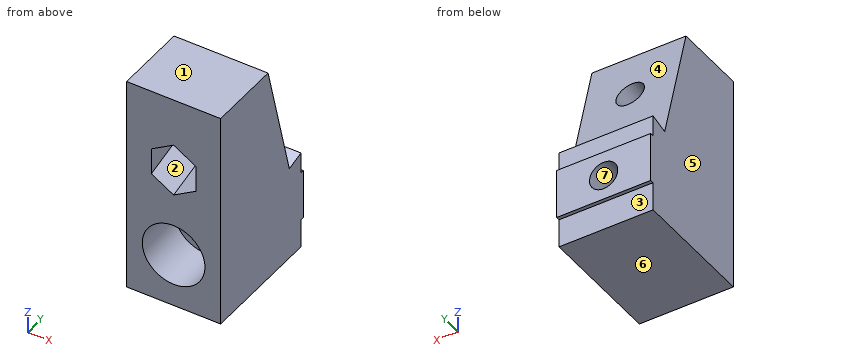
from build123d import *

# Parameters (mm, degrees)
BOSS_EXTRUDE1_DEPTH = 7.5
SKETCH2_R           = 2.25
CUT_EXTRUDE1_DEPTH  = 28.200078529
SKETCH3_R           = 2.25
CUT_EXTRUDE2_DEPTH  = 29.587584718
CUT_EXTRUDE3_START  = -4
CUT_EXTRUDE3_DEPTH  = 24.200078529
SKETCH5_W           = 15
SKETCH5_H           = 8
SKETCH5_R           = 2.25
BOSS_EXTRUDE2_DEPTH = 0.6
SKETCH6_R           = 5
CUT_EXTRUDE4_DEPTH  = 8


with BuildPart() as part:
    # Sketch1 → Boss-Extrude1 (new, symmetric)
    with BuildSketch(Plane(origin=(0, 0, 0), x_dir=(0, 0, -1), z_dir=(1, 0, 0))):
        Polygon((0.776457135, -2.897777479), (-19, -8.196863197), (-19, -20), (16, -20), (16, 0), (0, 0), align=None)
    extrude(amount=BOSS_EXTRUDE1_DEPTH, both=True)

    # Sketch2 → Cut-Extrude1 (cut, through all)
    with BuildSketch(Plane(origin=(0, -2.897777479, -0.776457135), x_dir=(1, 0, 0), z_dir=(0, 0.9659258262890682, 0.2588190451025216))):
        with Locations(Location((0, -12.003847577, 0), (0, 0, 270))):
            Circle(SKETCH2_R)
    extrude(amount=-CUT_EXTRUDE1_DEPTH, mode=Mode.SUBTRACT)

    # Sketch3 → Cut-Extrude2 (cut, through all)
    with BuildSketch(Plane.XZ.offset(20)):
        with Locations(Location((0, -7.39, 0), (0, 0, 270))):
            Circle(SKETCH3_R)
    extrude(amount=-CUT_EXTRUDE2_DEPTH, mode=Mode.SUBTRACT)

    # Sketch4 → Cut-Extrude3 (cut, through all)
    with BuildSketch(Plane(origin=(0, -2.897777479, -0.776457135), x_dir=(1, 0, 0), z_dir=(0, 0.9659258262890681, 0.2588190451025216)).offset(CUT_EXTRUDE3_START)):
        Polygon((0, -16.103034489), (3.55, -14.053441033), (3.55, -9.954254122), (0, -7.904660666), (-3.55, -9.954254122), (-3.55, -14.053441033), align=None)
    extrude(amount=-CUT_EXTRUDE3_DEPTH, mode=Mode.SUBTRACT)

    # Sketch5 → Boss-Extrude2 (add)
    with BuildSketch(Plane(origin=(0, 0, 0), x_dir=(1, 0, 0), z_dir=(0, 1, 0))):
        with Locations((0, 7.39)):
            Rectangle(SKETCH5_W, SKETCH5_H)
        with Locations(Location((0, 7.39, 0), (0, 0, 90))):
            Circle(SKETCH5_R, mode=Mode.SUBTRACT)
    extrude(amount=BOSS_EXTRUDE2_DEPTH)

    # Sketch6 → Cut-Extrude4 (cut)
    with BuildSketch(Plane.XZ.offset(20)):
        with Locations(Location((0, -7.39, 0), (0, 0, 270))):
            Circle(SKETCH6_R)
    extrude(amount=-CUT_EXTRUDE4_DEPTH, mode=Mode.SUBTRACT)


solid = part.part
The model under review builds one solid part; all positions refer to its coordinate system, in mm. Face numbers are marked on the shaded views. A direction names the side the tool comes from. Coordinates: 2 decimals unless noted, no trailing zeros. Write each loop counter-clockwise with the first axis right and the second up, starting at its lowest first coordinate (ties: lowest second). Pieces come first, ordered by that corner, then holes. Notation, with made-up numbers: (7.25, -2.75) - (34.25, -2.75) arc R27 cw to (34.25, 13.25) - close; hole circle Ø6 at (74.25, 28.25). An arc over 180 degrees is marked (long way). Answer as a JSON object with one key per item and string values. Group by question number.
1. Machinability: for the marked faces 1, 2 and 3, which of the approach directions +Z, -Z, +X, -X, +Y, -Y give a long, thin tool a straight path to every point of the face, cutting with its end or side? Answer none if there is none.
2. Add section D-D (y = -16.25). Give the boundary of the cut face in (x, z), plus the area to 3 significant figures.
3. To check wall thickness, follow probe 1 along X at (y, z) = (-11.75, 10); probe 2 along X at (y, z) = (-7.25, -7.39); probe 3 along Z at (x, y) = (-0.75, -18.5). State the ranges of each line that lie inside material, in increasing order.
4. Add section A-A (z = -7.39). Give the boundary of the cut face in (x, y).
5. Add section C-C (x = -5.75). Give the boundary of the cut face in (y, z), plus the area to 3 significant figures.
6. Clearance check with flat-ended pins moving along their axes: pin 1 Ø1.7 at (x, z) = (-1, -2) entering from +Y; pin 2 Ø3 at (x, z) = (0.5, -8.5) entering from -Y; pin 3 Ø1.5 at (x, z) = (0.5, -6.5) entering from -Y. State where each tip first meets the part, or that it passes through.
7. Add section B-B (x = 1.25). Give the boundary of the cut face in (y, z).
8. Mouldability with a two-part tool opening along Z and no side actions: class the marked faces 4, 5, 6 and 7 as pulls with the +Z half, pulls with the -Z half, needs draft (parallel to the pull), parting line crosses it, or undercut.
Findings:
{
 "1": {"face 1": "+Z, +X, -X, +Y, -Y", "face 2": "-Y", "face 3": "-Z, +X, -X, +Y"},
 "2": {"outline": "(-7.5, -16) - (7.5, -16) - (7.5, 19) - (-7.5, 19) - close; hole circle Ø10 at (0, -7.39); hole (-3.55, 5.95) - (0, 3.83) - (3.55, 5.95) - (3.55, 10.2) - (0, 12.32) - (-3.55, 10.2) - close", "area": "401 mm²"},
 "3": {"probe 1": "-7.5 to -3.55, 3.55 to 7.5", "probe 2": "-7.5 to -2.25, 2.25 to 7.5", "probe 3": "-16 to -12.33, -2.45 to 3.67, 11.27 to 19"},
 "4": {"outline": "(-7.5, -20) - (-5, -20) - (-5, -12) - (-2.25, -12) - (-2.25, 0.6) - (-7.5, 0.6) - close; (2.25, -12) - (5, -12) - (5, -20) - (7.5, -20) - (7.5, 0.6) - (2.25, 0.6) - close"},
 "5": {"outline": "(-20, -16) - (0, -16) - (0, -11.39) - (0.6, -11.39) - (0.6, -3.39) - (0, -3.39) - (0, 0) - (-2.9, -0.78) - (-8.2, 19) - (-20, 19) - close", "area": "596 mm²"},
 "6": {"pin 1": "y = 0", "pin 2": "y = -12", "pin 3": "through"},
 "7": {"outline": "(-20, -16) - (0, -16) - (0, -11.39) - (0.6, -11.39) - (0.6, -9.26) - (-12, -9.26) - (-12, -12.23) - (-20, -12.23) - close; (-20, -2.55) - (-12, -2.55) - (-12, -5.52) - (0.6, -5.52) - (0.6, -3.39) - (0, -3.39) - (0, 0) - (-2.9, -0.78) - (-5.52, 9.01) - (-9.38, 7.98) - (-8.99, 6.52) - (-20, 3.57) - close; (-20, 10.56) - (-10.74, 13.05) - (-10.35, 11.59) - (-6.49, 12.63) - (-8.2, 19) - (-20, 19) - close"},
 "8": {"face 4": "pulls with the +Z half", "face 5": "needs draft", "face 6": "pulls with the -Z half", "face 7": "undercut"}
}
